Work out the finished part from the listing and answer in its coordinate system (mm). Give positions to 0.01 mm unless a question says otherwise; leave off trailing zeros. One line per question, with ' | ' between items. Start each with the question number.
1. Section A-A (z = 4) is taken. Give the number of separate pieces and of enclosed holes in the cut face, plus the area to 3 significant figures.
2. Find the intervals of material crossed by line 1 (X direction, y = 215, z = 2.95); line 2 (Y direction, x = 290, z = 1.5); line 3 (Y direction, x = 30, z = 2.4), in increasing order.
3. Each of these flat-tipped pins is pushed along its axis until it touches: pin 1 (4 mm diameter, centred on x = 30, y = 215, fed in from -Z); pin 2 (1.5 mm diameter, centred on y = 252, z = 2.5, fed in from -X); pin 3 (1.5 mm diameter, centred on x = 260.5, z = 2, fed in from +Y); pin 4 (1.5 mm diameter, centred on x = 3, z = 2.5, fed in from +Y). Where does it stop, or does it pass through?
from build123d import *

# Parameters (mm, degrees)
SKIZZE1_R                       = 1.6
AUFSATZ_LINEAR_AUSTRAGEN1_DEPTH = 5


with BuildPart() as part:
    # Skizze1 → Aufsatz-Linear austragen1 (new body)
    with BuildSketch(Plane.XY):
        Polygon((5, 10), (5, 20), (0, 20), (0, 30), (5, 30), (5, 40), (0, 40), (0, 50), (5, 50), (5, 60), (0, 60), (0, 70), (5, 70), (5, 80), (0, 80), (0, 90), (5, 90), (5, 100), (0, 100), (0, 110), (5, 110), (5, 120), (0, 120), (0, 130), (5, 130), (5, 140), (0, 140), (0, 150), (5, 150), (5, 160), (0, 160), (0, 170), (5, 170), (5, 180), (0, 180), (0, 190), (5, 190), (5, 200), (0, 200), (0, 210), (5, 210), (5, 220), (35, 250), (45, 250), (45, 255), (55, 255), (55, 250), (65, 250), (65, 255), (75, 255), (75, 250), (85, 250), (85, 255), (95, 255), (95, 250), (105, 250), (105, 255), (115, 255), (115, 250), (125, 250), (125, 255), (135, 255), (135, 250), (145, 250), (145, 255), (155, 255), (155, 250), (165, 250), (165, 255), (175, 255), (175, 250), (185, 250), (185, 255), (195, 255), (195, 250), (205, 250), (205, 255), (215, 255), (215, 250), (225, 250), (225, 255), (235, 255), (235, 250), (245, 250), (245, 255), (255, 255), (255, 250), (265, 250), (265, 255), (275, 255), (275, 250), (305, 220), (305, 210), (310, 210), (310, 200), (305, 200), (305, 190), (310, 190), (310, 180), (305, 180), (305, 170), (310, 170), (310, 160), (305, 160), (305, 150), (310, 150), (310, 140), (305, 140), (305, 130), (310, 130), (310, 120), (305, 120), (305, 110), (310, 110), (310, 100), (305, 100), (305, 90), (310, 90), (310, 80), (305, 80), (305, 70), (310, 70), (310, 60), (305, 60), (305, 50), (310, 50), (310, 40), (305, 40), (305, 30), (310, 30), (310, 20), (305, 20), (305, 10), (310, 10), (310, 0), (305, 0), (5, 0), (0, 0), (0, 10), align=None)
        with Locations((20, 215)):
            Circle(SKIZZE1_R, mode=Mode.SUBTRACT)
        with Locations((30, 215)):
            Circle(SKIZZE1_R, mode=Mode.SUBTRACT)
        with Locations((290, 215)):
            Circle(SKIZZE1_R, mode=Mode.SUBTRACT)
        with Locations((280, 215)):
            Circle(SKIZZE1_R, mode=Mode.SUBTRACT)
        with Locations((20, 36)):
            Circle(SKIZZE1_R, mode=Mode.SUBTRACT)
        with Locations((155, 36)):
            Circle(SKIZZE1_R, mode=Mode.SUBTRACT)
        with Locations((290, 36)):
            Circle(SKIZZE1_R, mode=Mode.SUBTRACT)
    extrude(amount=AUFSATZ_LINEAR_AUSTRAGEN1_DEPTH)


solid = part.part
Conclusion:
1) separate pieces: 1 | enclosed holes: 7 | area: 75,700 mm²
2) line 1: 5 to 18.4, 21.6 to 28.4, 31.6 to 278.4, 281.6 to 288.4, 291.6 to 305 | line 2: 0 to 34.4, 37.6 to 213.4, 216.6 to 235 | line 3: 0 to 213.4, 216.6 to 245
3) pin 1: z = 0 | pin 2: x = 45 | pin 3: y = 250 | pin 4: y = 210
